from build123d import *

# Parameters (mm, degrees)
F0_W     = 57.15
F0_H     = 31.75
F1_DEPTH = 38.1
F3_DEPTH = 12.7
F5_DEPTH = 12.7
F7_DEPTH = 25.401


with BuildPart() as f1:
    # F0 (on Front) → F1 (new body)
    with BuildSketch(Plane.XZ):
        with Locations((28.575, 15.875)):
            Rectangle(F0_W, F0_H)
    extrude(amount=F1_DEPTH)

    # F2 (on face) → F3 (cut)
    with BuildSketch(Plane.XZ.offset(38.1)):
        Polygon((57.15, 31.75), (19.05, 31.75), (28.575, 0), (57.15, 0), align=None)
    extrude(amount=-F3_DEPTH, mode=Mode.SUBTRACT)

    # F4 (on face) → F5 (cut)
    with BuildSketch(Plane(origin=(0, 0, 0), x_dir=(-1, 0, 0), z_dir=(0, 1, 0))):
        Polygon((-28.575, 0), (-18.9710725099, 31.75), (-57.15, 31.75), (-57.15, 0), align=None)
    extrude(amount=-F5_DEPTH, mode=Mode.SUBTRACT)

    # F6 (on face) → F7 (cut, through all)
    with BuildSketch(Plane.XZ.offset(25.4)):
        Polygon((44.45, 31.75), (57.15, 0), (57.15, 31.75), align=None)
    extrude(amount=-F7_DEPTH, mode=Mode.SUBTRACT)


solid = f1.part
Work out the finished part from the listing and answer in its coordinate system (mm). A direction names the side the tool comes from. Coordinates: 2 decimals unless noted, no trailing zeros. Order: outer loops, then holes, each group sorted by start corner. A loop starts at its lowest first (then second) coordinate and runs counter-clockwise, first axis right, second up. Notation, with made-up numbers: (38.25, 49.5) - (83.25, 49.5) arc R19 cw to (83.25, 74.5) - close; hole circle Ø7 at (14, 10.5). An arc over 180 degrees is marked (long way). Put each result on its own line as item: value. Start each with the question number.
1) Find section D-D (y = -29). Give the vertices of the cut face in (x, z) (3 decimals).
2) Flat-ended cylindrical pins translate along their axes: pin 1 (10 mm diameter, centred on x = 13.5, z = 27.5, fed in from +Y); pin 2 (3 mm diameter, centred on y = -10, z = 8, fed in from +X); pin 3 (12 mm diameter, centred on x = 34, z = 28.5, fed in from -Y). Find the tip coordinate at first contact, or state that the pin passes through.
3) Find section C-C (x = 24.5). Give the vertices of the cut face in (y, z).
4) For faces 1 (the flat face through (11, -38.1, 16)), 2 (the flat face through (23.746, -31.839, 16.097)), 3 (the flat face through (38, -12.7, 16)), determine the directions among +Z, -Z, +X, -X, +Y, -Y from which every point of the face is accessible in a straight line to the end or side of a thin tool.
5) Find section A-A (z = 30). Give the vertices of the cut face in (x, y) (3 decimals).
6) Find section B-B (y = -13.5). Give the vertices of the cut face in (x, z), plus the area to 3 significant figures.
7) Find the intervals of material crossed by line 1 (Y direction, x = 35, z = 5.5); line 2 (X direction, y = -18, z = 12); line 3 (X direction, y = -31.5, z = 25.5) (3 decimals), in increasing order. Write a range as from..to.
Results list:
1. outline: (0, 0) - (28.575, 0) - (19.05, 31.75) - (0, 31.75) - close
2. pin 1: stops at y = 0
2. pin 2: stops at x = 26.61
2. pin 3: stops at y = -25.4
3. outline: (-38.1, 0) - (0, 0) - (0, 13.47) - (-12.7, 13.47) - (-12.7, 31.75) - (-25.4, 31.75) - (-25.4, 13.58) - (-38.1, 13.58) - close
4. face 1: +Z, -Z, +X, -X, -Y
4. face 2: +Z, +X, -Y
4. face 3: +Z, +X, +Y
5. outline: (0, -38.1) - (19.575, -38.1) - (19.575, -25.4) - (45.15, -25.4) - (45.15, -12.7) - (19.5, -12.7) - (19.5, 0) - (0, 0) - close
6. outline: (0, 0) - (57.15, 0) - (44.45, 31.75) - (0, 31.75) - close
6. area: 1,610 mm^2
7. line 1: y = -25.4..-12.7
7. line 2: x = 0..52.35
7. line 3: x = 0..20.925
